CAD build for the part. Positions are in the model's coordinates, mm. A direction names the side the tool comes from. Coordinates: 2 decimals unless noted, no trailing zeros.
from build123d import *

# Parameters (mm, degrees)
F1_DEPTH = 10
F3_DEPTH = 25
F4_R     = 5
F5_W     = 10
F5_H     = 10
F6_DEPTH = 25
F7_R     = 3
F8_SIZE  = 1


with BuildPart() as f1:
    # F0 (on Top) → F1 (new body)
    with BuildSketch(Plane.XY):
        Polygon((-10.9047358856, 5), (-1.6377953812, 5), (-6.2712656334, 21.0524187982), align=None)
        Polygon((0.893718563, 5), (10.1606590673, 5), (5.5271888152, 21.0524187982), align=None)
        with BuildLine():
            ThreePointArc((-25, -5), (0, -30), (25, -5))
            Line((25, -5), (-25, -5))
        make_face()
        with BuildLine():
            ThreePointArc((7.7540047355, 28.767107745), (8.969264738, 28.3356441964), (10.1606590673, 27.842088506))
            Line((10.1606590673, 27.842088506), (10.1606590673, 37.1048375964))
            Line((10.1606590673, 37.1048375964), (7.7540047355, 28.767107745))
        make_face()
        with BuildLine():
            Line((0.893718563, 37.1048375964), (0.893718563, 29.9840202355))
            ThreePointArc((0.893718563, 29.9840202355), (1.9468556818, 29.9240797815), (2.9965268036, 29.8197668626))
            Line((2.9965268036, 29.8197668626), (0.893718563, 37.1048375964))
        make_face()
        with BuildLine():
            ThreePointArc((-3.7711526138, 29.713931455), (-2.7069683761, 29.8530143486), (-1.6377953812, 29.9462948409))
            Line((-1.6377953812, 29.9462948409), (-1.6377953812, 37.1048375964))
            Line((-1.6377953812, 37.1048375964), (-3.7711526138, 29.713931455))
        make_face()
        with BuildLine():
            Line((-10.9047358856, 37.1048375964), (-10.9047358856, 27.4963716022))
            ThreePointArc((-10.9047358856, 27.4963716022), (-9.6819154679, 28.0490891983), (-8.4311989498, 28.535396412))
            Line((-8.4311989498, 28.535396412), (-10.9047358856, 37.1048375964))
        make_face()
        with BuildLine():
            ThreePointArc((21.1545569723, 18.3223391079), (24.0194080309, 11.9331117001), (25, 5))
            Line((25, 5), (25, 37.1048375964))
            Line((25, 37.1048375964), (20.3665297478, 21.0524187982))
            Line((20.3665297478, 21.0524187982), (21.1545569723, 18.3223391079))
        make_face()
        with BuildLine():
            Line((21.1545569723, 18.3223391079), (25, 5))
            ThreePointArc((25, 5), (24.0194080309, 11.9331117001), (21.1545569723, 18.3223391079))
        make_face()
        with BuildLine():
            ThreePointArc((15.7330594957, 24.4286087743), (18.0294324279, 22.3187634179), (20.0452738513, 19.9394443078))
            Line((20.0452738513, 19.9394443078), (20.3665297478, 21.0524187982))
            Line((20.3665297478, 21.0524187982), (15.7330594957, 37.1048375964))
            Line((15.7330594957, 37.1048375964), (15.7330594957, 24.4286087743))
        make_face()
        with BuildLine():
            Line((2.9965268036, 29.8197668626), (5.5271888152, 21.0524187982))
            Line((5.5271888152, 21.0524187982), (7.7540047355, 28.767107745))
            ThreePointArc((7.7540047355, 28.767107745), (5.4009725881, 29.4096189053), (2.9965268036, 29.8197668626))
        make_face()
        with BuildLine():
            Line((-8.4311989498, 28.535396412), (-6.2712656334, 21.0524187982))
            Line((-6.2712656334, 21.0524187982), (-3.7711526138, 29.713931455))
            ThreePointArc((-3.7711526138, 29.713931455), (-6.1295662271, 29.2369226155), (-8.4311989498, 28.535396412))
        make_face()
        with BuildLine():
            Line((-20.3665297478, 21.0524187982), (-20.0452738513, 19.9394443078))
            ThreePointArc((-20.0452738513, 19.9394443078), (-18.0294324279, 22.3187634179), (-15.7330594957, 24.4286087743))
            Line((-15.7330594957, 24.4286087743), (-15.7330594957, 37.1048375964))
            Line((-15.7330594957, 37.1048375964), (-20.3665297478, 21.0524187982))
        make_face()
        with BuildLine():
            Line((-25, 37.1048375964), (-25, 5))
            ThreePointArc((-25, 5), (-24.0194080309, 11.9331117001), (-21.1545569723, 18.3223391079))
            Line((-21.1545569723, 18.3223391079), (-20.3665297478, 21.0524187982))
            Line((-20.3665297478, 21.0524187982), (-25, 37.1048375964))
        make_face()
        with BuildLine():
            ThreePointArc((-21.1545569723, 18.3223391079), (-24.0194080309, 11.9331117001), (-25, 5))
            Line((-25, 5), (-21.1545569723, 18.3223391079))
        make_face()
        with BuildLine():
            Line((10.1606590673, 5), (15.7330594957, 5))
            Line((15.7330594957, 5), (15.7330594957, 24.4286087743))
            ThreePointArc((15.7330594957, 24.4286087743), (13.0588715525, 26.3182052194), (10.1606590673, 27.842088506))
            Line((10.1606590673, 27.842088506), (10.1606590673, 5))
        make_face()
        with BuildLine():
            Line((-1.6377953812, 5), (0.893718563, 5))
            Line((0.893718563, 5), (0.893718563, 29.9840202355))
            ThreePointArc((0.893718563, 29.9840202355), (-0.3725162805, 29.9972244783), (-1.6377953812, 29.9462948409))
            Line((-1.6377953812, 29.9462948409), (-1.6377953812, 5))
        make_face()
        with BuildLine():
            Line((-15.7330594957, 24.4286087743), (-15.7330594957, 5))
            Line((-15.7330594957, 5), (-10.9047358856, 5))
            Line((-10.9047358856, 5), (-10.9047358856, 27.4963716022))
            ThreePointArc((-10.9047358856, 27.4963716022), (-13.4069320833, 26.1010467066), (-15.7330594957, 24.4286087743))
        make_face()
        with BuildLine():
            ThreePointArc((20.0452738513, 19.9394443078), (20.615777266, 19.1417724391), (21.1545569723, 18.3223391079))
            Line((21.1545569723, 18.3223391079), (20.3665297478, 21.0524187982))
            Line((20.3665297478, 21.0524187982), (20.0452738513, 19.9394443078))
        make_face()
        with BuildLine():
            Line((15.7330594957, 24.4286087743), (15.7330594957, 5))
            Line((15.7330594957, 5), (20.0452738513, 19.9394443078))
            ThreePointArc((20.0452738513, 19.9394443078), (18.0294324279, 22.3187634179), (15.7330594957, 24.4286087743))
        make_face()
        with BuildLine():
            Line((-20.0452738513, 19.9394443078), (-15.7330594957, 5))
            Line((-15.7330594957, 5), (-15.7330594957, 24.4286087743))
            ThreePointArc((-15.7330594957, 24.4286087743), (-18.0294324279, 22.3187634179), (-20.0452738513, 19.9394443078))
        make_face()
        with BuildLine():
            Line((-20.3665297478, 21.0524187982), (-21.1545569723, 18.3223391079))
            ThreePointArc((-21.1545569723, 18.3223391079), (-20.615777266, 19.1417724391), (-20.0452738513, 19.9394443078))
            Line((-20.0452738513, 19.9394443078), (-20.3665297478, 21.0524187982))
        make_face()
        with BuildLine():
            Line((15.7330594957, 5), (25, 5))
            Line((25, 5), (21.1545569723, 18.3223391079))
            ThreePointArc((21.1545569723, 18.3223391079), (20.615777266, 19.1417724391), (20.0452738513, 19.9394443078))
            Line((20.0452738513, 19.9394443078), (15.7330594957, 5))
        make_face()
        with BuildLine():
            Line((5.5271888152, 21.0524187982), (10.1606590673, 5))
            Line((10.1606590673, 5), (10.1606590673, 27.842088506))
            ThreePointArc((10.1606590673, 27.842088506), (8.969264738, 28.3356441964), (7.7540047355, 28.767107745))
            Line((7.7540047355, 28.767107745), (5.5271888152, 21.0524187982))
        make_face()
        with BuildLine():
            Line((0.893718563, 29.9840202355), (0.893718563, 5))
            Line((0.893718563, 5), (5.5271888152, 21.0524187982))
            Line((5.5271888152, 21.0524187982), (2.9965268036, 29.8197668626))
            ThreePointArc((2.9965268036, 29.8197668626), (1.9468556818, 29.9240797815), (0.893718563, 29.9840202355))
        make_face()
        with BuildLine():
            Line((-6.2712656334, 21.0524187982), (-1.6377953812, 5))
            Line((-1.6377953812, 5), (-1.6377953812, 29.9462948409))
            ThreePointArc((-1.6377953812, 29.9462948409), (-2.7069683761, 29.8530143486), (-3.7711526138, 29.713931455))
            Line((-3.7711526138, 29.713931455), (-6.2712656334, 21.0524187982))
        make_face()
        with BuildLine():
            Line((-10.9047358856, 27.4963716022), (-10.9047358856, 5))
            Line((-10.9047358856, 5), (-6.2712656334, 21.0524187982))
            Line((-6.2712656334, 21.0524187982), (-8.4311989498, 28.535396412))
            ThreePointArc((-8.4311989498, 28.535396412), (-9.6819154679, 28.0490891983), (-10.9047358856, 27.4963716022))
        make_face()
        Polygon((25, -5), (25, 5), (15.7330594957, 5), (10.1606590673, 5), (0.893718563, 5), (-1.6377953812, 5), (-10.9047358856, 5), (-15.7330594957, 5), (-25, 5), (-25, -5), align=None)
        with BuildLine():
            Line((-21.1545569723, 18.3223391079), (-25, 5))
            Line((-25, 5), (-15.7330594957, 5))
            Line((-15.7330594957, 5), (-20.0452738513, 19.9394443078))
            ThreePointArc((-20.0452738513, 19.9394443078), (-20.615777266, 19.1417724391), (-21.1545569723, 18.3223391079))
        make_face()
    extrude(amount=F1_DEPTH)

    # F2 (on face) → F3 (cut)
    with BuildSketch(Plane.XY.offset(10)):
        with BuildLine():
            ThreePointArc((0.3781150769, 1.944110059), (0.8106415831, 3.5947742399), (0.9562301539, 5.2949434623))
            ThreePointArc((0.9562301539, 5.2949434623), (0.8106415831, 6.9951126847), (0.3781150769, 8.6457768657))
            ThreePointArc((0.3781150769, 8.6457768657), (-0.2, 5.2949434623), (0.3781150769, 1.944110059))
        make_face()
        with BuildLine():
            ThreePointArc((0.3781150769, 8.6457768657), (0.8106415831, 6.9951126847), (0.9562301539, 5.2949434623))
            ThreePointArc((0.9562301539, 5.2949434623), (0.8106415831, 3.5947742399), (0.3781150769, 1.944110059))
            ThreePointArc((0.3781150769, 1.944110059), (11.5001692224, -4.5594679668), (19.8, 5.2949434623))
            ThreePointArc((19.8, 5.2949434623), (11.5001692224, 15.1493548915), (0.3781150769, 8.6457768657))
        make_face()
        with BuildLine():
            ThreePointArc((0.3781150769, 1.944110059), (-0.2, 5.2949434623), (0.3781150769, 8.6457768657))
            ThreePointArc((0.3781150769, 8.6457768657), (-19.0437698461, 5.2949434623), (0.3781150769, 1.944110059))
        make_face()
    extrude(amount=-F3_DEPTH, mode=Mode.SUBTRACT)

    # F4
    f4_edges = [f1.edges().sort_by_distance(p)[0] for p in [
        (0.378115, 8.645777, 5),
        (0.378115, 1.94411, 5),
    ]]
    fillet(f4_edges, radius=F4_R)

    # F5 (on face) → F6 (cut)
    with BuildSketch(Plane.XY.offset(10)):
        with Locations((0, -17.2223318368)):
            Rectangle(F5_W, F5_H)
    extrude(amount=-F6_DEPTH, mode=Mode.SUBTRACT)

    # F7
    f7_edges = [f1.edges().sort_by_distance(p)[0] for p in [
        (-5, -22.222332, 5),
        (-5, -12.222332, 5),
        (5, -12.222332, 5),
        (5, -22.222332, 5),
    ]]
    fillet(f7_edges, radius=F7_R)

    # F8
    f8_edges = [f1.edges().sort_by_distance(p)[0] for p in [
        (0, -30, 10),
        (0, -30, 0),
        (-19.04377, 5.294943, 10),
        (0, -12.222332, 10),
        (0, -22.222332, 0),
        (0.378115, -1.376735, 0),
    ]]
    chamfer(f8_edges, length=F8_SIZE)


solid = f1.part
1) Which spindle directions (+Z, -Z, +X, -X, +Y, -Y) get a long thin tool onto all of the face, cutting with end or side? Do faces 1 (the conical face through (-4.297, -21.57, 9.285)), 2 (the flat face through (-5, -17, 5)), 3 (the flat face through (22.716, 29.191, 4.93)). Say none if no direction does.
2) Two-plate mould, pull along Y, no slides. Class faces 4 (the conical face through (-0.532, -29.168, 0.174)), 5 (the conical face through (4.34, -12.94, 0.73)), 6 (the cylindrical face through (5.434, 29.402, 4.93)): released by +Y, released by -Y, zero draft, split by the parting line, or undercut.
3) Slice it at A-A (z = 6.25). Give the number of separate pieces and of enclosed holes in the cut face, plus the area to 3 significant figures.
4) Drill centre lines: probe 1 along Y at (x, z) = (-5.5, 6.25); probe 2 along Y at (x, z) = (-15, 6.25); probe 3 along X at (y, z) = (0.5, 2.25). Where is each one in solid material? Low to high.
5) Pin check, flat tips, straight feed: P1, Ø6, axis at x = 8.5, z = 6, coming from the -Y side; P2, Ø1.2, axis at x = 1, z = 4.5, coming from the +Y side; P3, Ø3, axis at y = -17.5, z = 7, coming from the +X side. Stop position of each tip, or through.
Worked out:
1. face 1: +Z
1. face 2: +Z, -Z
1. face 3: +Z, -Z, +Y
2. face 4: released by -Y
2. face 5: undercut
2. face 6: released by +Y
3. separate pieces: 1
3. enclosed holes: 2
3. area: 1,970 mm2
4. probe 1: y = -29.39 to -4.06, 14.65 to 29.39
4. probe 2: y = -25 to -2.74, 13.33 to 25
4. probe 3: x = -25 to -17.82, 18.58 to 25
5. P1: stops at y = -29.39
5. P2: stops at y = 37.1
5. P3: stops at x = 22.45
